Input: part model. Units: mm. Frame: model coordinates. Coordinates: 2 decimals unless noted, no trailing zeros. Order: outer loops, then holes, each group sorted by start corner. A loop starts at its lowest first (then second) coordinate and runs counter-clockwise, first axis right, second up. Notation, with made-up numbers: (2, 8.25) -> (50, 8.25) arc R4 ccw to (50, 14.25) -> close; hole circle Ø10 at (-38.5, 20). An arc over 180 degrees is marked (long way). Use one line per item in the form item = value. Start each with the question number.
1) Section query A-A on x = 112.5. Output: boundary loops of the cut face in (y, z).
2) Ray query, line 1 along Z through (x, y) = (167, 0.4); line 2 along Z through (x, y) = (54.5, 3.1); line 3 along Z through (x, y) = (163.5, 3.2). Return the intervals inside material, ascending.
3) Pin query (flat end, axial travel): pin 1 (6.5 mm diameter, centred on x = 118.1, z = 135.75, fed in from -Y); pin 2 (2 mm diameter, centred on y = 1.5, z = 101, fed in from -X). Return the tip coordinate at first contact, or that it passes through.
4) Section query B-B on y = 2.9. Count the separate pieces of the cut face and the enclosed holes in it, then the cut area to 3 significant figures.
from build123d import *

# Parameters (mm, degrees)
ESQUISSE1_R        = 1.5
ESQUISSE1_R_2      = 1
ESQUISSE1_R_3      = 2
BOSS_EXTRU_1_DEPTH = 4


with BuildPart() as part:
    # Esquisse1 → Boss.-Extru.1 (new body)
    with BuildSketch(Plane(origin=(0, 0, 0), x_dir=(1, 0, 0), z_dir=(0, 1, 0))):
        with BuildLine():
            Line((20.099012054, -176.753119553), (180.099012054, -176.753119553))
            Line((180.099012054, -176.753119553), (180.099012054, -143.304210871))
            add(Edge.make_bspline(
                [(200.099012054, -5.402601665), (200.027324087, -10.863493838), (197.583796942, -30.094661829), (186.072485669, -54.954429671), (180.370262256, -81.651562253), (173.133805108, -108.569720083), (178.097171518, -129.349130809), (180.099012054, -143.304210871)],
                knots=[0.01165801, 0.01165801, 0.01165801, 0.01165801, 0.124408467, 0.420109799, 0.574806268, 0.697902863, 1, 1, 1, 1], degree=3))
            Line((200.099012054, -5.402601665), (200.099012054, 8.246880447))
            Line((200.099012054, 8.246880447), (0.099012054, 8.246880447))
            Line((0.099012054, 8.246880447), (0.099012054, -5.402601665))
            add(Edge.make_bspline(
                [(0.099012054, -5.402601665), (0.170700021, -10.863493838), (2.927056594, -30.094661829), (14.083581709, -54.954429671), (20.192714137, -81.651562253), (26.973296377, -108.569720083), (22.623790852, -129.349130809), (20.099012054, -143.304210871)],
                knots=[0.01165801, 0.01165801, 0.01165801, 0.01165801, 0.124408467, 0.420109799, 0.574806268, 0.697902863, 1, 1, 1, 1], degree=3))
            Line((20.099012054, -143.304210871), (20.099012054, -176.753119553))
        make_face()
        with Locations(Location((33.099012054, -145.753119553, 0), (0, 0, 270))):
            Circle(ESQUISSE1_R, mode=Mode.SUBTRACT)
        with Locations(Location((33.099012054, -162.753119553, 0), (0, 0, 270))):
            Circle(ESQUISSE1_R, mode=Mode.SUBTRACT)
        with Locations(Location((167.099012054, -162.753119553, 0), (0, 0, 90))):
            Circle(ESQUISSE1_R, mode=Mode.SUBTRACT)
        with Locations(Location((167.099012054, -145.753119553, 0), (0, 0, 90))):
            Circle(ESQUISSE1_R, mode=Mode.SUBTRACT)
        with Locations(Location((92.099012054, -46.753119553, 0), (0, 0, 270))):
            Circle(ESQUISSE1_R_2, mode=Mode.SUBTRACT)
        with Locations(Location((108.099012054, -46.753119553, 0), (0, 0, 270))):
            Circle(ESQUISSE1_R_2, mode=Mode.SUBTRACT)
        with Locations(Location((82.099012054, -171.753119553, 0), (0, 0, 270))):
            Circle(ESQUISSE1_R_3, mode=Mode.SUBTRACT)
        with Locations(Location((118.099012054, -135.753119553, 0), (0, 0, 270))):
            Circle(ESQUISSE1_R_3, mode=Mode.SUBTRACT)
        with Locations(Location((164.677408292, -55.946819434, 0), (0, 0, 270))):
            Circle(ESQUISSE1_R, mode=Mode.SUBTRACT)
        with Locations(Location((122.677408292, -55.946819434, 0), (0, 0, 270))):
            Circle(ESQUISSE1_R, mode=Mode.SUBTRACT)
        with Locations(Location((50.545382216, -71.701846064, 0), (0, 0, 270))):
            Circle(ESQUISSE1_R_3, mode=Mode.SUBTRACT)
        with Locations(Location((102.045382216, -118.201846064, 0), (0, 0, 270))):
            Circle(ESQUISSE1_R_3, mode=Mode.SUBTRACT)
        with BuildLine():
            Line((7.599012054, 2.246880447), (192.599012054, 2.246880447))
            ThreePointArc((192.599012054, 2.246880447), (194.599012054, 0.246880447), (192.599012054, -1.753119553))
            Line((192.599012054, -1.753119553), (7.599012054, -1.753119553))
            ThreePointArc((7.599012054, -1.753119553), (5.599012054, 0.246880447), (7.599012054, 2.246880447))
        make_face(mode=Mode.SUBTRACT)
        with BuildLine():
            Line((182, -7.753119553), (194, -7.753119553))
            ThreePointArc((194, -7.753119553), (196, -9.753119553), (194, -11.753119553))
            Line((194, -11.753119553), (182, -11.753119553))
            ThreePointArc((182, -11.753119553), (180, -9.753119553), (182, -7.753119553))
        make_face(mode=Mode.SUBTRACT)
        with BuildLine():
            Line((18.198024108, -7.753119553), (6.198024108, -7.753119553))
            ThreePointArc((6.198024108, -7.753119553), (4.198024108, -9.753119553), (6.198024108, -11.753119553))
            Line((6.198024108, -11.753119553), (18.198024108, -11.753119553))
            ThreePointArc((18.198024108, -11.753119553), (20.198024108, -9.753119553), (18.198024108, -7.753119553))
        make_face(mode=Mode.SUBTRACT)
        with BuildLine():
            Line((75.911540887, -57.098867648), (91.911540887, -57.098867648))
            ThreePointArc((91.911540887, -57.098867648), (94.411540887, -59.598867648), (91.911540887, -62.098867648))
            Line((91.911540887, -62.098867648), (75.911540887, -62.098867648))
            ThreePointArc((75.911540887, -62.098867648), (73.411540887, -59.598867648), (75.911540887, -57.098867648))
        make_face(mode=Mode.SUBTRACT)
    extrude(amount=BOSS_EXTRU_1_DEPTH)


solid = part.part
Answers below:
q1.outline = (0, -8.25) -> (4, -8.25) -> (4, -2.25) -> (0, -2.25) -> close; (0, 1.75) -> (4, 1.75) -> (4, 176.75) -> (0, 176.75) -> close
q2.line_1 = -8.25 to -2.25, 1.75 to 144.26, 147.25 to 161.26, 164.25 to 176.75
q2.line_2 = -8.25 to -2.25, 1.75 to 176.75
q2.line_3 = -8.25 to -2.25, 1.75 to 55.02, 56.88 to 176.75
q3.pin_1 = 0
q3.pin_2 = 24.06
q4.separate_pieces = 1
q4.enclosed_holes = 16
q4.area = 30,400 mm^2
